Input: dimensioned drawing with shaded views. Units: mm. Origin: part minimum x, y, z. Coordinates: 2 decimals unless noted, no trailing zeros. Loops run counter-clockwise (first coordinate to the right, second up) from the corner with the lowest first, then second, coordinate; pieces in that order, holes last. Notation, with made-up numbers: (38.25, 37) - (80.25, 37) arc R23 ccw to (80.25, 65) - close; hole circle Ø9 at (49.25, -15). An arc over 180 degrees is marked (long way). Put each result on its own line as item: value. Start each with the question number.
1) Section D-D on y = 2.35. Output: boundary loops of the cut face in (x, z).
2) Contact query for a flat-ended pin moving along its axis: pin 1 Ø1 at (x, y) = (2.5, 46) entering from +Z. Output: stop coordinate, or through.
3) Section C-C on z = 0.75. Output: boundary loops of the cut face in (x, y), and give its area (3 significant figures).
4) Material intervals for line 1 along Y through (x, z) = (3.5, 1.6); line 2 along Y through (x, z) = (3.5, 0.8); line 3 along Y through (x, z) = (4.5, 1.75), sorted ascending. Write a range as from..to.
5) Section B-B on y = 29. Output: boundary loops of the cut face in (x, z).
6) Section A-A on x = 3.5. Output: boundary loops of the cut face in (y, z).
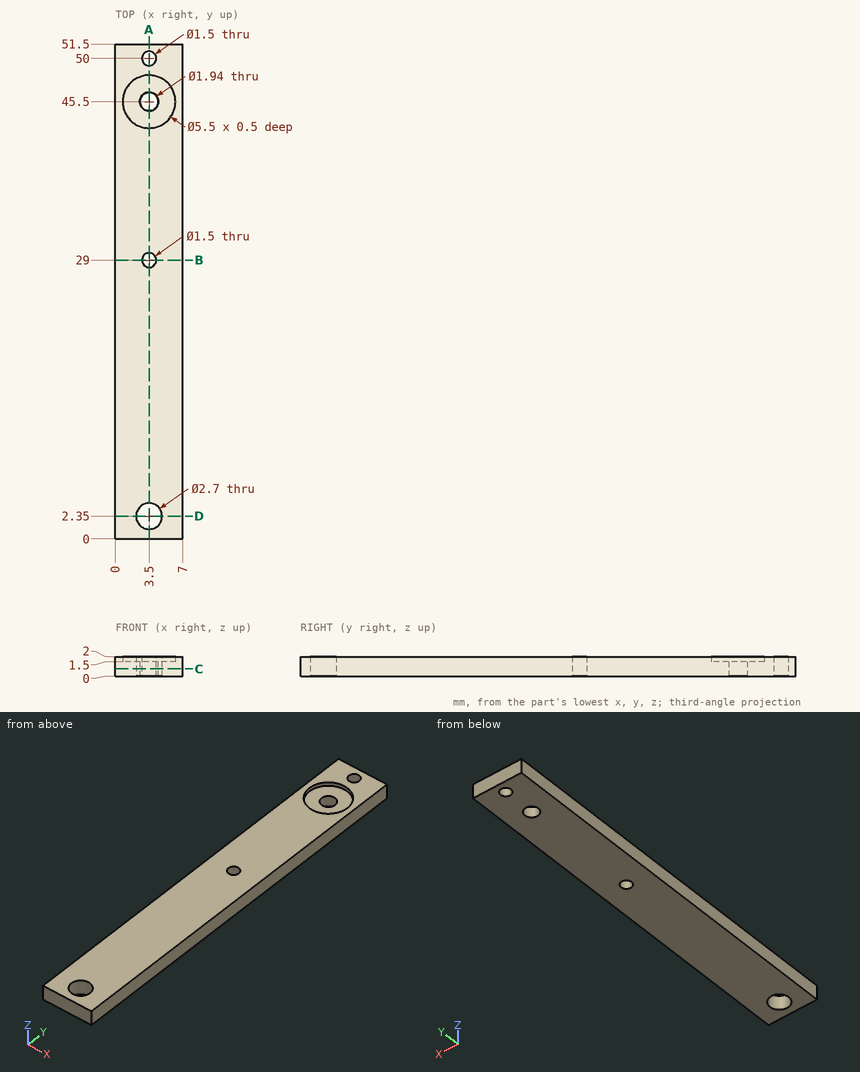
Answer block:
1. outline: (0, 0) - (2.15, 0) - (2.15, 2) - (0, 2) - close; (4.85, 0) - (7, 0) - (7, 2) - (4.85, 2) - close
2. pin 1: stops at z = 1.5
3. outline: (0, 0) - (7, 0) - (7, 51.5) - (0, 51.5) - close; hole circle Ø2.7 at (3.5, 2.35); hole circle Ø1.94 at (3.5, 45.5); hole circle Ø1.5 at (3.5, 29); hole circle Ø1.5 at (3.5, 50)
3. area: 348 mm²
4. line 1: y = 0..1, 3.7..28.25, 29.75..42.75, 48.25..49.25, 50.75..51.5
4. line 2: y = 0..1, 3.7..28.25, 29.75..44.53, 46.47..49.25, 50.75..51.5
4. line 3: y = 0..1.44, 3.26..42.94, 48.06..51.5
5. outline: (0, 0) - (2.75, 0) - (2.75, 2) - (0, 2) - close; (4.25, 0) - (7, 0) - (7, 2) - (4.25, 2) - close
6. outline: (0, 0) - (1, 0) - (1, 2) - (0, 2) - close; (3.7, 0) - (28.25, 0) - (28.25, 2) - (3.7, 2) - close; (29.75, 0) - (44.53, 0) - (44.53, 1.5) - (42.75, 1.5) - (42.75, 2) - (29.75, 2) - close; (46.47, 0) - (49.25, 0) - (49.25, 2) - (48.25, 2) - (48.25, 1.5) - (46.47, 1.5) - close; (50.75, 0) - (51.5, 0) - (51.5, 2) - (50.75, 2) - close
